from build123d import *

# Parameters (mm, degrees)
F0_R     = 20.1
F0_R_2   = 13.3
F0_R_3   = 12.1
F0_R_4   = 10
F1_DEPTH = 1
F2_DEPTH = 8
F3_W     = 5
F3_H     = 10
F3_W_2   = 10
F3_H_2   = 5
F4_DEPTH = 1.001


with BuildPart() as f1:
    # F0 (on Top) → F1 (new body)
    with BuildSketch(Plane.XY):
        Circle(F0_R)
        Circle(F0_R_2, mode=Mode.SUBTRACT)
        Circle(F0_R_2)
        Circle(F0_R_3, mode=Mode.SUBTRACT)
        Circle(F0_R_3)
        Circle(F0_R_4, mode=Mode.SUBTRACT)
    extrude(amount=F1_DEPTH)

    # F0 (on Top) → F2 (join)
    with BuildSketch(Plane.XY):
        Circle(F0_R_2)
        Circle(F0_R_3, mode=Mode.SUBTRACT)
    extrude(amount=F2_DEPTH)

    # F3 (on face) → F4 (cut, through all)
    with BuildSketch(Plane.XY.offset(1)):
        with Locations((0, 20.1)):
            Rectangle(F3_W, F3_H)
        Polygon((-8.909545443, 12.4450793489), (-15.9806132548, 19.5161471607), (-19.5161471607, 15.9806132548), (-12.4450793489, 8.909545443), align=None)
        with Locations((-20.1, 0)):
            Rectangle(F3_W_2, F3_H_2)
        Polygon((-12.4450793489, -8.909545443), (-19.5161471607, -15.9806132548), (-15.9806132548, -19.5161471607), (-8.909545443, -12.4450793489), align=None)
        with Locations((0, -20.1)):
            Rectangle(F3_W, F3_H)
        Polygon((8.909545443, -12.4450793489), (15.9806132548, -19.5161471607), (19.5161471607, -15.9806132548), (12.4450793489, -8.909545443), align=None)
        with Locations((20.1, 0)):
            Rectangle(F3_W_2, F3_H_2)
        Polygon((12.4450793489, 8.909545443), (19.5161471607, 15.9806132548), (15.9806132548, 19.5161471607), (8.909545443, 12.4450793489), align=None)
    extrude(amount=-F4_DEPTH, mode=Mode.SUBTRACT)


solid = f1.part
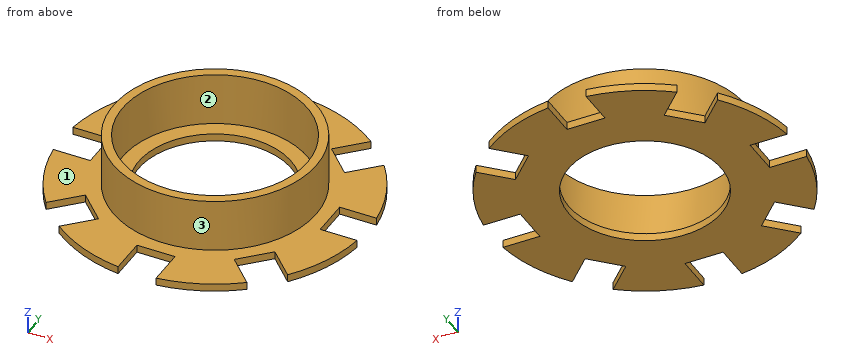
For this review, take the finished solid that the model builds, in its own axes (mm). Face numbers are marked on the shaded views. Round coordinates to 2 decimals unless told otherwise and drop trailing zeros. Write each loop counter-clockwise with the first axis right and the second up, starting at its lowest first coordinate (ties: lowest second). Pieces come first, ordered by that corner, then holes. Notation, with made-up numbers: (54, -20.5) -> (63, -20.5) arc R25 cw to (63, 4.5) -> close; hole circle Ø4 at (-2, 29.25). An arc over 180 degrees is marked (long way). Put each result on its own line as item: value.
Q1. To check wall thickness, follow L1, parallel to Y at x = 0, z = 5.25; L2, parallel to Y at x = 0, z = 0.4. State the ranges of each line that lie inside material, in increasing order. Write a range as [from, to].
Determined:
L1: y = [-13.3, -12.1], [12.1, 13.3]
L2: y = [-15.1, -10], [10, 15.1]
Q2. Consider section C-C on z = 2. State the section outline as (x, y) points, and give its area (3 significant figures).
Determined:
outline: circle Ø26.6 at (0, 0); hole circle Ø24.2 at (0, 0)
area: 95.8 mm^2
Q3. Consider section D-D on y = -16.5. State the section outline as (x, z) points, and give its area (3 significant figures).
Determined:
outline: (-11.48, 0) -> (-2.5, 0) -> (-2.5, 1) -> (-11.48, 1) -> close; (2.5, 0) -> (11.48, 0) -> (11.48, 1) -> (2.5, 1) -> close
area: 18.0 mm^2
Q4. Consider section A-A on x = 0. State the section outline as (y, z) points.
Determined:
outline: (-15.1, 0) -> (-10, 0) -> (-10, 1) -> (-12.1, 1) -> (-12.1, 8) -> (-13.3, 8) -> (-13.3, 1) -> (-15.1, 1) -> close; (10, 0) -> (15.1, 0) -> (15.1, 1) -> (13.3, 1) -> (13.3, 8) -> (12.1, 8) -> (12.1, 1) -> (10, 1) -> close
Q5. The part is to be moulded in two halves that separate along Y. For the marked faces 1, 2 and 3, say which applies: released by +Y, released by -Y, zero draft, split by the parting line, or undercut.
Determined:
face 1: zero draft
face 2: undercut
face 3: split by the parting line
Q6. Clearance check with flat-ended pins moving along their axes: pin 1 Ø4 at (x, z) = (-7.5, 5.5) entering from +Y; pin 2 Ø19.5 at (x, y) = (0.5, -3) entering from +Z; pin 3 Ø1.1 at (y, z) = (-0.5, 0.5) entering from +X; pin 4 Ø0.8 at (y, z) = (-17.5, 0.5) entering from -X. State where each tip first meets the part, or that it passes through.
Determined:
pin 1: stops at y = 12.11
pin 2: stops at z = 8
pin 3: stops at x = 15.1
pin 4: stops at x = -10.56
